Autodesk Inventor part; units mm, degrees
ref_plane "YZ Plane" through (0, 0, 0) normal (1, 0, 0) x (0, 1, 0)
ref_plane "XZ Plane" through (0, 0, 0) normal (0, 1, 0) x (-1, 0, 0)
ref_plane "XY Plane" through (0, 0, 0) normal (0, 0, 1) x (1, 0, 0)
sketch "Sketch1" plane through (0, 0, 0) normal (0, 1, 0) x (-1, 0, 0)
  line L0 (34.5, 64.5) -> (-34.5, 64.5)
  line L1 (-34.5, 64.5) -> (-34.5, -64.5)
  line L2 (-34.5, -64.5) -> (34.5, -64.5)
  line L3 (34.5, -64.5) -> (34.5, 64.5)
  line L4 (34.5, 64.5) -> (-34.5, -64.5) construction
  line L5 (-34.5, 64.5) -> (34.5, -64.5) construction
  point P0 (0, 0)
  dimension "d0" = 69
  dimension "d1" = 129
extrude "Extrusion1" add sketch "Sketch1" along normal blind 1.8
sketch "Sketch2" plane through (0, 1.8, 0) normal (0, 1, 0) x (1, 0, 0)
  line L0 (-29, -52) -> (29, -52)
  line L1 (29, -52) -> (29, 52)
  line L2 (29, 52) -> (-29, 52)
  line L3 (-29, 52) -> (-29, -52)
  line L4 (-29, -52) -> (29, 52) construction
  line L5 (29, -52) -> (-29, 52) construction
  point P0 (0, 0)
  dimension "d4" = 104
  dimension "d5" = 58
extrude "Extrusion2" cut sketch "Sketch2" against normal up to next
sketch "Sketch3" plane through (0, 1.8, 0) normal (0, 1, 0) x (1, 0, 0)
  line L0 (34.5, 64.5) -> (-34.5, 64.5)
  line L1 (-34.5, 64.5) -> (34.5, 64.5)
  line L2 (34.5, 64.5) -> (34.5, -64.5)
  line L3 (34.5, -64.5) -> (-34.5, -64.5)
  line L4 (-34.5, -64.5) -> (-34.5, 64.5)
  line L5 (-32.5, 62.5) -> (32.5, 62.5)
  line L6 (32.5, 62.5) -> (32.5, -62.5)
  line L7 (32.5, -62.5) -> (-32.5, -62.5)
  line L8 (-32.5, -62.5) -> (-32.5, 62.5)
  point P0 (0, 0)
  dimension "d8" = 2
  dimension "d9" = 2
  dimension "d10" = 2
  dimension "d11" = 2
extrude "Extrusion3" add sketch "Sketch3" along normal blind 20
sketch "Sketch4" plane through (0, 1.8, 0) normal (0, 1, 0) x (1, 0, 0)
  line L0 (32.5, -62.5) -> (-32.5, -62.5)
  line L1 (-32.5, 62.5) -> (-32.5, -62.5)
  line L2 (32.5, -62.5) -> (-32.5, -62.5)
  line L3 (-32.5, -62.5) -> (-32.5, -55)
  line L4 (-32.5, -55) -> (32.5, -55)
  line L5 (32.5, -55) -> (32.5, -62.5)
  line L6 (32.5, 62.5) -> (-32.5, 62.5)
  dimension "d36" = 117.5
extrude "Extrusion4" add sketch "Sketch4" along normal blind 3
sketch "Sketch5" plane through (0, 1.8, 0) normal (0, 1, 0) x (1, 0, 0)
  line L0 (-32.5, -62.5) -> (-32.5, 62.5)
  line L1 (-32.5, -62) -> (32.5, -62)
  line L2 (32.5, 62.5) -> (32.5, -62.5)
  line L3 (29, -52) -> (-29, -52)
  point P0 (0, 0)
  dimension "d17" = 10
fillet "Fillet1" radius 3 8 edges at (-32.5, 13.3, 62.5) (-34.5, 10.9, 64.5) (34.5, 10.9, 64.5) (32.5, 13.3, 62.5) (-32.5, 11.8, -62.5) (32.5, 11.8, -62.5) (34.5, 10.9, -64.5) (-34.5, 10.9, -64.5)
fillet "Fillet2" radius 2 8 edges at (33.6213, 0, -63.6213) (0, 0, -64.5) (-33.6213, 0, -63.6213) (-34.5, 0, 0) (-33.6213, 0, 63.6213) (0, 0, 64.5) (33.6213, 0, 63.6213) (34.5, 0, 0)
sketch "Sketch6" plane through (-34.5, 21.8, -61.5) normal (-1, 0, 0) x (0, 0, 1)
  line L0 (6.5, -12) -> (6.5, -15)
  line L1 (6.5, -15) -> (6.5, -12)
  line L2 (103, -12.7) -> (111, -12.7)
  line L3 (112, -13.7) -> (112, -15.3)
  line L4 (111, -16.3) -> (103, -16.3)
  line L5 (102, -15.3) -> (102, -13.7)
  line L6 (9.5, -20) -> (113.5, -20)
  line L7 (113.5, -20) -> (9.5, -20)
  line L8 (116.5, -20) -> (2, -20)
  line L9 (2, -20) -> (116.5, -20)
  arc A0 (103, -12.7) -> (102, -13.7) centre (103, -13.7) ccw
  arc A1 (102, -15.3) -> (103, -16.3) centre (103, -15.3) ccw
  arc A2 (112, -13.7) -> (111, -12.7) centre (111, -13.7) ccw
  arc A3 (111, -16.3) -> (112, -15.3) centre (111, -15.3) ccw
  line L10 (2, -20) -> (-1, -20)
  line L11 (-1, -20) -> (2, -20)
  line L12 (116.5, -20) -> (116.5, -17)
  point P0 (61.5, -21.8)
  point P1 (102, -12.7)
  point P2 (112, -16.3)
  point P3 (112, -12.7)
  point P4 (121, -15)
  point P5 (112, -14.5)
  point P6 (107, -16.3)
  dimension "d20" = 10
  dimension "d21" = 3.6
  dimension "d25" = 1
  dimension "d38" = 4.5
  dimension "d39" = 3.7
extrude "Extrusion5" cut sketch "Sketch6" against normal up to next
sketch "Sketch7" plane through (34.5, 21.8, 61.5) normal (1, 0, 0) x (0, 0, -1)
  line L0 (116.5, -12) -> (116.5, -15)
  line L1 (6.5, -20) -> (121, -20)
  circle A0 centre (35.5, -15.5) radius 1.5
  line L2 (6.5, -20) -> (6.5, -17)
  point P0 (61.5, -21.8)
  point P1 (2, -15)
  point P2 (6.5, -18.5)
  dimension "d29" = 4.5
  dimension "d30" = 3
  dimension "d37" = 29
extrude "Extrusion6" cut sketch "Sketch7" against normal up to next
pattern_linear "Rectangular Pattern1" count 5 spacing 7.3 along (0, 0, -1) of "Extrusion6"
sketch "Sketch8" plane through (0, 0, 0) normal (0, -1, 0) x (1, 0, 0)
  point P0 (0, 0)
sketch "Sketch9" plane through (-34.5, 21.8, -61.5) normal (-1, 0, 0) x (0, 0, 1)
  line L0 (123, 0) -> (0, 0)
  line L1 (14, 0) -> (18, 0)
  line L2 (18, 0) -> (18, -0.75)
  line L3 (18, -0.75) -> (14, -0.75)
  line L4 (14, -0.75) -> (14, 0)
  point P0 (61.5, -21.8)
  point P1 (-1, 0)
  point P2 (14, -0.375)
  point P3 (18, 0)
  dimension "d40" = 0.75
  dimension "d41" = 4
  dimension "d42" = 15
extrude "Extrusion7" cut sketch "Sketch9" against normal up to surface (2 mm away)
fillet "Fillet3" radius 0.5 5 edges at (0, 21.8, 62.5) (-32.5, 21.8, 8) (0, 21.8, -62.5) (-32.5, 21.8, -53.5) (32.5, 21.8, 0)
sketch "Sketch10" plane through (-29.5, 1.8, -62.5) normal (0, 0, 1) x (1, 0, 0)
  line L0 (-3.2949, 5.75) -> (63.1479, 5.75)
  line L1 (63.1479, 5.75) -> (63.1479, 4.25)
  line L2 (63.1479, 4.25) -> (-3.2949, 4.25)
  line L3 (-3.2949, 4.25) -> (-3.2949, 5.75)
  line L4 (59, 0) -> (0, 0)
  line L5 (7, 5.75) -> (7, 4.25)
  line L6 (52, 5.75) -> (52, 4.25)
  line L7 (-3, 19.5) -> (-3, 0)
  line L8 (62, 0) -> (62, 19.5)
  point P0 (29.5, -1.8)
  point P1 (52, 5)
  point P2 (62, 4.25)
  point P3 (62, 5.75)
  point P4 (-3, 5.75)
  point P5 (-3, 4.25)
  dimension "d46" = 4.25
  dimension "d47" = 1.5
  dimension "d48" = 10
  dimension "d49" = 10
extrude "Extrusion8" add sketch "Sketch10" along normal blind 6 contours L5 L2 L7 L0 | L0 L8 L2 L6
fillet "Fillet4" radius 5 2 edges at (-22.5, 6.8, -56.5) (22.5, 6.8, -56.5)
Read the model definition and answer for the solid it produces. Units are mm, in the model's axes. A direction names the side the tool comes from. Coordinates: 2 decimals unless noted, no trailing zeros. Write each loop counter-clockwise with the first axis right and the second up, starting at its lowest first coordinate (ties: lowest second). Pieces come first, ordered by that corner, then holes. Notation, with made-up numbers: (64, -35.75) -> (95, -35.75) arc R25 cw to (95, -23.75) -> close; hole circle Ø3 at (81.25, 21). An arc over 180 degrees is marked (long way). Write item = value, one per line.
(1) Section C-C on x = -20.5 is taken. Write down the section's boundary in (y, z), plus the area to 3 significant figures.
From the geometry:
outline = (0, -62.5) arc R2 ccw to (2, -64.5) -> (21.8, -64.5) -> (21.8, -63) arc R0.5 ccw to (21.3, -62.5) -> (1.8, -62.5) -> (1.8, -52) -> (0, -52) -> close; (0, 52) -> (1.8, 52) -> (1.8, 55) -> (4.8, 55) -> (4.8, 62.5) -> (21.3, 62.5) arc R0.5 ccw to (21.8, 63) -> (21.8, 64.5) -> (2, 64.5) arc R2 ccw to (0, 62.5) -> close
area = 146 mm2
(2) Section B-B on z = -16.5 is taken. Write down the section's boundary in (x, y).
From the geometry:
outline = (-34.5, 2) arc R2 ccw to (-32.5, 0) -> (-29, 0) -> (-29, 1.8) -> (-32.5, 1.8) -> (-32.5, 21.3) arc R0.5 ccw to (-33, 21.8) -> (-34.5, 21.8) -> close; (29, 0) -> (32.5, 0) arc R2 ccw to (34.5, 2) -> (34.5, 21.8) -> (33, 21.8) arc R0.5 ccw to (32.5, 21.3) -> (32.5, 1.8) -> (29, 1.8) -> close
(3) For a pull along Y with two mould halves and no side action, classify faces 4 (the face through (31, 0, 0)), 5 (the face through (24, 6.79, -57.93)), 6 (the face through (33.51, 7.31, 27.11)) as +Y half, -Y half, draft (parallel to the pull), parting line (faces both ways), or undercut.
From the geometry:
face_4 = -Y half
face_5 = draft
face_6 = undercut
(4) Which of the six approach directions +Z, -Z, +X, -X, +Y, -Y give full straight-line access (tool end or side, diameter ignored) to faces 1 (the face through (33.514, 7.787, 18.895)), 2 (the face through (-28, 7.55, -60)), 3 (the face through (28, 6.05, -60))?
From the geometry:
face_1 = +X
face_2 = +Y
face_3 = none
(5) Given pin 1 Ø3 at (x, z) = (-26.5, -58.5) entering from -Y; pin 2 Ø0.9 at (y, z) = (1, -1) entering from +X; pin 3 Ø6 at (x, z) = (-15.5, 59) entering from +Y; pin 4 Ø5 at (x, z) = (28.5, -59) entering from +Y, each flat-ended and moving along its own axis, determine where each tip first touches the part or whether it passes through.
From the geometry:
pin_1 = 0
pin_2 = 34.42
pin_3 = 4.8
pin_4 = 7.55
(6) Section D-D on y = 18 is taken. Write down the section's boundary in (x, z), plus the area to 3 significant figures.
From the geometry:
outline = (-34.5, -61.5) arc R3 ccw to (-31.5, -64.5) -> (31.5, -64.5) arc R3 ccw to (34.5, -61.5) -> (34.5, 61.5) arc R3 ccw to (31.5, 64.5) -> (-31.5, 64.5) arc R3 ccw to (-34.5, 61.5) -> close; hole (-32.5, -59.5) arc R3 ccw to (-29.5, -62.5) -> (29.5, -62.5) arc R3 ccw to (32.5, -59.5) -> (32.5, 59.5) arc R3 ccw to (29.5, 62.5) -> (-29.5, 62.5) arc R3 ccw to (-32.5, 59.5) -> close
area = 776 mm2
(7) Straight lines are drawn through the part: L1, parallel to X at y = 16.75, z = -35.5; L2, parallel to Z at x = -16.5, y = 11.5; L3, parallel to Y at x = 12, z = 56.5. For each, find the intervals that lie inside material, in ascending order. Write a range as from..to.
From the geometry:
L1 = -34.5..-32.5, 32.5..34.5
L2 = -64.5..-62.5, 62.5..64.5
L3 = 0..4.8
(8) Section A-A on z = 18.7 is taken. Write down the section's boundary in (x, y), plus the area to 3 significant figures.
From the geometry:
outline = (-34.5, 2) arc R2 ccw to (-32.5, 0) -> (-29, 0) -> (-29, 1.8) -> (-32.5, 1.8) -> (-32.5, 21.3) arc R0.5 ccw to (-33, 21.8) -> (-34.5, 21.8) -> close; (29, 0) -> (32.5, 0) arc R2 ccw to (34.5, 2) -> (34.5, 4.8) -> (32.5, 4.8) -> (32.5, 1.8) -> (29, 1.8) -> close; (32.5, 7.8) -> (34.5, 7.8) -> (34.5, 21.8) -> (33, 21.8) arc R0.5 ccw to (32.5, 21.3) -> close
area = 92.0 mm2
